For this review, take the finished solid that the model builds, in its own axes (mm). A direction names the side the tool comes from. Coordinates: 2 decimals unless noted, no trailing zeros. Write each loop counter-clockwise with the first axis right and the second up, starting at its lowest first coordinate (ties: lowest second). Pieces come first, ordered by that corner, then holes. Notation, with made-up numbers: M 31.5,-5 L 56.5,-5 A22 cw 56.5,22 Z; hole C 67.5,77.25 d3. An arc over 180 degrees is marked long. One line per question, with ' | ' between items.
from build123d import *

# Parameters (mm, degrees)
F1_DEPTH = 78


with BuildPart() as f1:
    # F0 (on Front) → F1 (new body)
    with BuildSketch(Plane.XZ):
        with BuildLine():
            Line((0, 15), (0, 0))
            Line((0, 0), (150, 0))
            Line((150, 0), (150, 15))
            Line((150, 15), (131.919114, 15))
            Line((131.919114, 15), (131.919114, 53.964467))
            ThreePointArc((131.919114, 53.964467), (77.582593, 113.941463), (18.039792, 59.129489))
            Line((18.039792, 59.129489), (18.039792, 54.870511))
            Line((18.039792, 54.870511), (18.039792, 15))
            Line((18.039792, 15), (0, 15))
        make_face()
        with BuildLine():
            ThreePointArc((115, 57), (103.284271, 28.715729), (75, 17))
            ThreePointArc((75, 17), (35, 57), (75, 97))
            ThreePointArc((75, 97), (103.284271, 85.284271), (115, 57))
        make_face(mode=Mode.SUBTRACT)
    extrude(amount=F1_DEPTH)


solid = f1.part
1) We need section B-B on y = -54. State the section outline as (x, z) points, then the cut area to 3 significant figures.
Responses:
outline: M 0,0 L 150,0 L 150,15 L 131.92,15 L 131.92,53.96 A57 ccw long 18.04,59.13 L 18.04,15 L 0,15 Z; hole M 75,17 A40 ccw 115,57 A40 ccw long Z | area: 7,110 mm^2
2) Machinability: for faces 1 (the flat face through (9, -38, 15)), 2 (the flat face through (150, -38, 7)), which of the approach directions +Z, -Z, +X, -X, +Y, -Y give a long, thin tool a straight path to every point of the face, cutting with its end or side? Answer none if there is none.
Responses:
face 1: +Z, -X, +Y, -Y | face 2: +Z, -Z, +X, +Y, -Y
3) Insertion check: pin 1 Ø22 at (y, z) = (-24.5, 45.5) entering from -X; pin 2 Ø1.5 at (y, z) = (-32.5, 46.5) entering from +X; pin 3 Ø9 at (x, y) = (6, -26) entering from +Z. Each pin has a flat end and moves straight along its axis. Give the tip position at first contact, or say it passes through.
Responses:
pin 1: x = 18.04 | pin 2: x = 131.92 | pin 3: z = 15
4) We need section C-C on x = 100.5. State the section outline as (y, z) points, then the cut area to 3 significant figures.
Responses:
outline: M -78,0 L 0,0 L 0,26.18 L -78,26.18 Z; M -78,87.82 L 0,87.82 L 0,107.98 L -78,107.98 Z | area: 3,610 mm^2
5) To check wall thickness, follow line 1 along X through (y, z) = (-73, 31.5); line 2 along Z through (x, y) = (69, -55); line 3 along X through (y, z) = (-27, 66.5). State the ranges of each line that lie inside material, in increasing order. Write a range as [from, to].
Responses:
line 1: [18.04, 44.18], [105.82, 131.92] | line 2: [0, 17.45], [96.55, 113.68] | line 3: [18.8, 36.14], [113.86, 131.2]
6) We need section A-A on z = 33. State the section outline as (x, y) points, then the cut area to 3 significant figures.
Responses:
outline: M 18.04,-78 L 43,-78 L 43,0 L 18.04,0 Z; M 107,-78 L 131.92,-78 L 131.92,0 L 107,0 Z | area: 3,890 mm^2
